Design review of the part built by this model. Coordinates are the model's own, in mm. A direction names the side the tool comes from. Give positions to 0.01 mm unless a question says otherwise; leave off trailing zeros. Order: outer loops, then holes, each group sorted by start corner. A loop starts at its lowest first (then second) coordinate and runs counter-clockwise, first axis right, second up. Notation, with made-up numbers: (28, -0.5) -> (53, -0.5) arc R28 ccw to (53, 36.5) -> close; hole circle Ø4 at (9, 39.25). An arc over 180 degrees is marked (long way). One line per item, written item: value.
Solid Edge part; units mm, degrees
sketch "Sketch1" plane through (0, 0, 0) normal (0, -1, 0) x (1, 0, 0)
  line L0 (275, 20) -> (275, 350)
  line L1 (275, 350) -> (-75, 350)
  line L2 (-75, 350) -> (-75, 20)
  line L3 (-75, 20) -> (0, 20)
  line L4 (0, 20) -> (0, 0)
  line L5 (0, 0) -> (200, 0)
  line L6 (200, 0) -> (200, 20)
  line L7 (200, 20) -> (275, 20)
extrude "Protrusion1" add sketch "Sketch1" against normal blind 20
hole "Bohrung_1" at (70, 0, 40) direction (0, 1, 0) diameter 10.5 end up to next start chamfer 1 start chamfer angle 45
hole "Hole1" at (130, 0, 40) direction (0, 1, 0) diameter 10.5 end up to next start chamfer 1 start chamfer angle 45
hole "Hole2" at (130, 0, 170) direction (0, 1, 0) diameter 10.5 end up to next start chamfer 1 start chamfer angle 45
hole "Hole3" at (70, 0, 170) direction (0, 1, 0) diameter 10.5 end up to next start chamfer 1 start chamfer angle 45
Item 1: Clearance check with flat-ended pins moving along their axes: P1, Ø6.5, axis at x = 70, z = 170, coming from the -Y side; P2, Ø1.5, axis at x = -23, y = 2.5, coming from the -Z side. State where each tip first meets the part, or that it passes through.
Returned:
P1: through
P2: z = 20
Item 2: Draft analysis for pull direction Z (two halves, no side actions). For faces 4 (the flat face through (-38, 10, 20)), 5 (the flat face through (102, 10, 350)), 6 (the cylindrical face through (64.875, 10.367, 41.138)), state which applies: pulls with the +Z half, pulls with the -Z half, needs draft (parallel to the pull), parting line crosses it, or undercut.
Returned:
face 4: pulls with the -Z half
face 5: pulls with the +Z half
face 6: undercut
Item 3: Add section D-D on x = 215.5. Give the boundary of the cut face in (y, z), plus the area to 3 significant figures.
Returned:
outline: (0, 20) -> (20, 20) -> (20, 350) -> (0, 350) -> close
area: 6,600 mm²
Item 4: Machinability: for faces 1 (the flat face through (237, 10, 20)), 2 (the flat face through (0, 10, 10)), 3 (the flat face through (275, 10, 183)), which of the approach directions +Z, -Z, +X, -X, +Y, -Y give a long, thin tool a straight path to every point of the face, cutting with its end or side? Answer none if there is none.
Returned:
face 1: -Z, +X, +Y, -Y
face 2: -Z, -X, +Y, -Y
face 3: +Z, -Z, +X, +Y, -Y
Item 5: Add section B-B on y = 5. Give the boundary of the cut face in (x, z).
Returned:
outline: (-75, 20) -> (0, 20) -> (0, 0) -> (200, 0) -> (200, 20) -> (275, 20) -> (275, 350) -> (-75, 350) -> close; hole circle Ø10.5 at (70, 40); hole circle Ø10.5 at (70, 170); hole circle Ø10.5 at (130, 40); hole circle Ø10.5 at (130, 170)
Item 6: Add section A-A on z = 40. Give the boundary of the cut face in (x, y).
Returned:
outline: (-75, 0) -> (63.75, 0) -> (64.75, 1) -> (64.75, 20) -> (-75, 20) -> close; (75.25, 1) -> (76.25, 0) -> (123.75, 0) -> (124.75, 1) -> (124.75, 20) -> (75.25, 20) -> close; (135.25, 1) -> (136.25, 0) -> (275, 0) -> (275, 20) -> (135.25, 20) -> close
Item 7: Add section C-C on x = 70. Give the boundary of the cut face in (y, z).
Returned:
outline: (0, 0) -> (20, 0) -> (20, 34.75) -> (1, 34.75) -> (0, 33.75) -> close; (0, 46.25) -> (1, 45.25) -> (20, 45.25) -> (20, 164.75) -> (1, 164.75) -> (0, 163.75) -> close; (0, 176.25) -> (1, 175.25) -> (20, 175.25) -> (20, 350) -> (0, 350) -> close
Item 8: To check wall thickness, follow line 1 along Z through (x, y) = (70, 5); line 2 along Z through (x, y) = (259, 2.25); line 3 along X through (y, z) = (12, 44.5). State the ranges of each line that lie inside material, in increasing order. Write a range as from..to.
Returned:
line 1: 0..34.75, 45.25..164.75, 175.25..350
line 2: 20..350
line 3: -75..67.3, 72.7..127.3, 132.7..275
